from build123d import *

# Parameters (mm, degrees)
SKETCH_1_W             = 426
SKETCH_1_H             = 55.7
SM_BASE_FLANGE_1_DEPTH = 1.5
SM_EDGE_FLANGE_2_DEPTH = 55.7
SM_EDGE_FLANGE_3_DEPTH = 426
SM_EDGE_FLANGE_4_DEPTH = 55.7
SKETCH_25_W            = 15
SKETCH_25_H            = 15
CUT_EXTRUDE_1_DEPTH    = 16
SKETCH_26_W            = 15
SKETCH_26_H            = 15
CUT_EXTRUDE_2_DEPTH    = 16
SKETCH_27_R            = 2.25
CUT_EXTRUDE_3_DEPTH    = 433.860820588


# Sheet-metal steps are written as plain solids
with BuildPart() as part:
    # Sketch 1 → Базовая кромка1 (new body)
    with BuildSketch(Plane.XY):
        with Locations((213, 27.85)):
            Rectangle(SKETCH_1_W, SKETCH_1_H)
    extrude(amount=-SM_BASE_FLANGE_1_DEPTH)

    # Ребро-кромка2 section (across the edge) → Ребро-кромка2 (add)
    with BuildSketch(Plane(origin=(-1.5, 0, -1.5), x_dir=(1, 0, 0), z_dir=(0, 1, 0))):
        with BuildLine():
            Line((-1.5, 1.5), (-1.5, 13.5))
            Line((-1.5, 13.5), (0, 13.5))
            Line((0, 13.5), (0, 1.5))
            ThreePointArc((0, 1.5), (0.439339828, 0.439339828), (1.5, 0))
            Line((1.5, 0), (1.5, -1.5))
            ThreePointArc((1.5, -1.5), (-0.621320344, -0.621320344), (-1.5, 1.5))
        make_face()
    extrude(amount=SM_EDGE_FLANGE_2_DEPTH)

    # Ребро-кромка3 section (across the edge) → Ребро-кромка3 (add)
    with BuildSketch(Plane(origin=(426, -1.5, -1.5), x_dir=(0, 1, 0), z_dir=(-1, 0, 0))):
        with BuildLine():
            Line((-1.5, 1.5), (-1.5, 13.5))
            Line((-1.5, 13.5), (0, 13.5))
            Line((0, 13.5), (0, 1.5))
            ThreePointArc((0, 1.5), (0.439339828, 0.439339828), (1.5, 0))
            Line((1.5, 0), (1.5, -1.5))
            ThreePointArc((1.5, -1.5), (-0.621320344, -0.621320344), (-1.5, 1.5))
        make_face()
    extrude(amount=SM_EDGE_FLANGE_3_DEPTH)

    # Ребро-кромка4 section (across the edge) → Ребро-кромка4 (add)
    with BuildSketch(Plane(origin=(427.5, 55.7, -1.5), x_dir=(-1, 0, 0), z_dir=(0, -1, 0))):
        with BuildLine():
            Line((-1.5, 1.5), (-1.5, 13.5))
            Line((-1.5, 13.5), (0, 13.5))
            Line((0, 13.5), (0, 1.5))
            ThreePointArc((0, 1.5), (0.439339828, 0.439339828), (1.5, 0))
            Line((1.5, 0), (1.5, -1.5))
            ThreePointArc((1.5, -1.5), (-0.621320344, -0.621320344), (-1.5, 1.5))
        make_face()
    extrude(amount=SM_EDGE_FLANGE_4_DEPTH)

    # Эскиз25 → Вырез-Вытянуть1 (cut)
    with BuildSketch(Plane.ZY.offset(3)):
        with Locations((-7.5, 48.2)):
            Rectangle(SKETCH_25_W, SKETCH_25_H)
    extrude(amount=-CUT_EXTRUDE_1_DEPTH, mode=Mode.SUBTRACT)

    # Эскиз26 → Вырез-Вытянуть2 (cut)
    with BuildSketch(Plane(origin=(429, 0, 0), x_dir=(0, 0, -1), z_dir=(1, 0, 0))):
        with Locations((7.5, 48.2)):
            Rectangle(SKETCH_26_W, SKETCH_26_H)
    extrude(amount=-CUT_EXTRUDE_2_DEPTH, mode=Mode.SUBTRACT)

    # Эскиз27 → Вырез-Вытянуть3 (cut, through all)
    with BuildSketch(Plane.XY):
        with Locations((39, 48.7)):
            Circle(SKETCH_27_R)
        with Locations((387, 48.7)):
            Circle(SKETCH_27_R)
    extrude(amount=-CUT_EXTRUDE_3_DEPTH, mode=Mode.SUBTRACT)


solid = part.part
The listing builds one solid part. Answer for the finished solid, in the listing's coordinates (mm). A direction names the side the tool comes from. Coordinates: 2 decimals unless noted, no trailing zeros. Write each loop counter-clockwise with the first axis right and the second up, starting at its lowest first coordinate (ties: lowest second). Pieces come first, ordered by that corner, then holes. Notation, with made-up numbers: M -4,44 L 50,44 A12 ccw 50,63 Z; hole C 73,-23 d5. An arc over 180 degrees is marked long. Put each result on its own line as item: value. Start each with the question number.
1. Flat-ended cylindrical pins translate along their axes: P1, Ø3, axis at x = 61.5, y = 32.5, coming from the -Z side; P2, Ø2.5, axis at y = -1.5, z = -4, coming from the -X side; P3, Ø4, axis at x = 387, y = 48.7, coming from the +Z side; P4, Ø5, axis at x = 39, y = 48.7, coming from the +Z side. Find the tip coordinate at first contact, or state that the pin passes through.
2. For a pull along X with two mould halves and no side action, classify faces 4 (the flat face through (427.5, 21, -9)), 5 (the flat face through (216, -1.5, -9)), 6 (the flat face through (210, 28, -1.5)), 7 (the flat face through (429, 21, -9)) as pulls with the +X half, pulls with the -X half, needs draft (parallel to the pull), parting line crosses it, or undercut.
3. Consider line 1 (X direction, y = 16, z = -6.25); line 2 (X direction, y = 47.5, z = -1); line 3 (Y direction, x = 387, z = -0.45). Determine where each line is inside the solid, lowest interval first. Write a range as from..to.
4. Which of the six approach directions +Z, -Z, +X, -X, +Y, -Y give full straight-line access (tool end or side, diameter ignored) to faces 1 (the flat face through (-1.5, 20, -9)), 2 (the flat face through (2, 40.7, -1)), 3 (the flat face through (424, 40.7, -1))?
5. A cutting plane is placed at B-B on y = 11.5. Write down the section's boundary in (x, z).
6. A cutting plane is placed at C-C on x = 168.5. Write down the section's boundary in (y, z), then the cut area to 3 significant figures.
7. A cutting plane is placed at A-A on z = -11.25. Write down the section's boundary in (x, y).
Resolved:
1. P1: stops at z = -1.5
1. P2: stops at x = 0
1. P3: passes through
1. P4: stops at z = 0
2. face 4: undercut
2. face 5: needs draft
2. face 6: undercut
2. face 7: pulls with the +X half
3. line 1: x = -3..-1.5, 427.5..429
3. line 2: x = 13..37.1, 40.9..385.1, 388.9..413
3. line 3: y = -1.58..46.45, 50.95..55.7
4. face 1: -Z, +Y, -Y
4. face 2: +Z, -Z, -X, +Y
4. face 3: +Z, -Z, +X, +Y
5. outline: M -3,-15 L -1.5,-15 L -1.5,-3 A1.5 cw 0,-1.5 L 426,-1.5 A1.5 cw 427.5,-3 L 427.5,-15 L 429,-15 L 429,-3 A3 ccw 426,0 L 0,0 A3 ccw -3,-3 Z
6. outline: M -3,-15 L -1.5,-15 L -1.5,-3 A1.5 cw 0,-1.5 L 55.7,-1.5 L 55.7,0 L 0,0 A3 ccw -3,-3 Z
6. area: 107 mm2
7. outline: M -3,0 L -1.5,0 L -1.5,40.7 L -3,40.7 Z; M 0,-3 L 426,-3 L 426,-1.5 L 0,-1.5 Z; M 427.5,0 L 429,0 L 429,40.7 L 427.5,40.7 Z
